```python
from build123d import *

# Parameters (mm, degrees)
F1_DEPTH      = 76.2
F3_DEPTH      = 54.411857
F3_DEPTH_BACK = 50.8
F4_R          = 4.699
F5_DEPTH      = 32.667806


with BuildPart() as f1:
    # F0 (on Right) → F1 (new body)
    with BuildSketch(Plane.YZ):
        Polygon((-54.410857, -32.666806), (40.839143, -32.666806), (40.839143, -13.616806), (15.439143, -13.616806), (15.439143, 37.183194), (-9.960857, 37.183194), (-9.960857, -13.616806), (-54.410857, -13.616806), align=None)
    extrude(amount=F1_DEPTH)

    # F2 (on Front) → F3 (cut, two sides)
    with BuildSketch(Plane.XZ) as f3_sk:
        Polygon((52.712968, 8.363965), (52.712968, 36.938965), (52.712968, 49.710356), (23.8252, 49.710356), (23.8252, 36.769882), (23.8252, 8.194882), align=None)
    extrude(amount=F3_DEPTH, mode=Mode.SUBTRACT)
    extrude(f3_sk.sketch, amount=-F3_DEPTH_BACK, mode=Mode.SUBTRACT)

    # F4 (on Top) → F5 (cut, through all)
    with BuildSketch(Plane.XY):
        with Locations((12.7, 28.12115)):
            Circle(F4_R)
        with Locations((63.163701, 28.038393)):
            Circle(F4_R)
        with Locations((63.163701, -41.310414)):
            Circle(F4_R)
        with Locations((12.7, -41.310414)):
            Circle(F4_R)
    extrude(amount=-F5_DEPTH, mode=Mode.SUBTRACT)


solid = f1.part
```
Here's how the part is built. I have some questions about the finished solid (model axes, mm). A direction names the side the tool comes from. Give positions to 0.01 mm unless a question says otherwise; leave off trailing zeros. Write each loop counter-clockwise with the first axis right and the second up, starting at its lowest first coordinate (ties: lowest second). Pieces come first, ordered by that corner, then holes.
(1) Will these pins go through, and if not, where does the flat tip stop? pin 1 (15 mm diameter, centred on x = 51.5, z = 18.5, fed in from -Y); pin 2 (11 mm diameter, centred on x = 63.16, y = 28.04, fed in from +Z); pin 3 (10 mm diameter, centred on y = 28, z = -17.5, fed in from -X); pin 4 (2 mm diameter, centred on x = 22, z = -4, fed in from +Y).
Output values:
pin 1: stops at y = -9.96
pin 2: stops at z = -13.62
pin 3: stops at x = 0
pin 4: stops at y = 15.44
(2) Imagine slicing it at C-C, the plane y = 26.5. Write out the boundary of the cut face in (x, z), and give its area (3 significant figures).
Output values:
outline: (0, -32.67) - (8.29, -32.67) - (8.29, -13.62) - (0, -13.62) - close; (17.11, -32.67) - (58.72, -32.67) - (58.72, -13.62) - (17.11, -13.62) - close; (67.6, -32.67) - (76.2, -32.67) - (76.2, -13.62) - (67.6, -13.62) - close
area: 1,110 mm2
(3) On a 3-axis mill with a long thin cutter (end or side, diameter ignored), from which of +Z, -Z, +X, -X, +Y, -Y can I reach the whole of each face in a straight line? I mean faces 1 (the face through (23.825, 3, 23)), 2 (the face through (38, -9.961, 6)), 3 (the face through (67.646, 29.45, -23.008)), 4 (the face through (38, 15.439, 6)). Say none if no direction works.
Output values:
face 1: +Z, +Y, -Y
face 2: +Z, +X, -X, -Y
face 3: +Z, -Z
face 4: +Z, +X, -X, +Y
(4) Imagine slicing it at A-A, the plane x = 12.7. Write out the boundary of the cut face in (y, z), and give its area (3 significant figures).
Output values:
outline: (-54.41, -32.67) - (-46.01, -32.67) - (-46.01, -13.62) - (-54.41, -13.62) - close; (-36.61, -32.67) - (23.42, -32.67) - (23.42, -13.62) - (15.44, -13.62) - (15.44, 37.18) - (-9.96, 37.18) - (-9.96, -13.62) - (-36.61, -13.62) - close; (32.82, -32.67) - (40.84, -32.67) - (40.84, -13.62) - (32.82, -13.62) - close
area: 2,750 mm2
(5) If I drill on L1, parallel to Y at x = 12.7, z = -26.25; L2, parallel to X at y = -2, z = 21; L3, parallel to Z at x = 32.5, y = 31.5, over which ranges is the centre line in solid material (lowest first)?
Output values:
L1: y = -54.41 to -46.01, -36.61 to 23.42, 32.82 to 40.84
L2: x = 0 to 23.83, 52.71 to 76.2
L3: z = -32.67 to -13.62
(6) Imagine slicing it at B-B, the plane z = 11.5. Write out the boundary of the cut face in (x, y).
Output values:
outline: (0, -9.96) - (23.83, -9.96) - (23.83, 15.44) - (0, 15.44) - close; (52.71, -9.96) - (76.2, -9.96) - (76.2, 15.44) - (52.71, 15.44) - close
(7) Imagine slicing it at D-D, the plane z = -28. Write out the boundary of the cut face in (x, y).
Output values:
outline: (0, -54.41) - (76.2, -54.41) - (76.2, 40.84) - (0, 40.84) - close; hole circle Ø9.4 at (12.7, -41.31); hole circle Ø9.4 at (12.7, 28.12); hole circle Ø9.4 at (63.16, -41.31); hole circle Ø9.4 at (63.16, 28.04)
(8) Thinking about a two-plate mould opening in X: for faces 5 (the face through (38, -7, -32.667)), 6 (the face through (65.69, -37.35, -23.01)), 7 (the face through (76.2, 3, -5)), which applies, pulls with the +X half, pulls with the -X half, needs draft (parallel to the pull), parting line crosses it, or undercut?
Output values:
face 5: needs draft
face 6: undercut
face 7: pulls with the +X half
